Read the model definition and answer for the solid it produces. Units are mm, in the model's axes. Face numbers are marked on the shaded views. A direction names the side the tool comes from. Give positions to 0.01 mm unless a question says otherwise; leave off trailing zeros. Loops run counter-clockwise (first coordinate to the right, second up) from the corner with the lowest first, then second, coordinate; pieces in that order, holes last. Notation, with made-up numbers: (-31, -31.75) -> (-21, -31.75) arc R14 cw to (-21, -21.75) -> close; hole circle Ø4 at (11.5, 76.5). An arc over 180 degrees is marked (long way). Write each question's results on one line, items separated by ' | '. Start each with the question number.
Item 1: Find the intervals of material crossed by line 1 (X direction, y = 23.6, z = 6); line 2 (X direction, y = 23.8, z = 6); line 3 (Y direction, x = -3, z = 9.75), in increasing order.
Item 2: Each of these flat-tipped pins is pushed along its axis until it touches: P1, Ø1.8, axis at x = -26, z = 6, coming from the -Y side; P2, Ø5.5, axis at x = -14.75, y = -19.5, coming from the -Z side; P3, Ø13, axis at y = 10.5, z = 3, coming from the +X side; P4, Ø11, axis at y = -12, z = 5.5, coming from the -X side. Where does it stop, or does it pass through?
Item 3: Section B-B on y = 6 is taken. Write down the section's boundary in (x, z), and give its area (3 significant figures).
Item 4: Section D-D on z = 6 is taken. Write down the section's boundary in (x, y), and give its area (3 significant figures).
Item 5: Section C-C on x = -26 is taken. Write down the section's boundary in (y, z), and give its area (3 significant figures).
Item 6: Which of the six approach directions +Z, -Z, +X, -X, +Y, -Y give full straight-line access (tool end or side, diameter ignored) to the marked faces 1, 2 and 3?
Item 7: Section A-A on z = 18 is taken. Write down the section's boundary in (x, y), and give its area (3 significant figures).
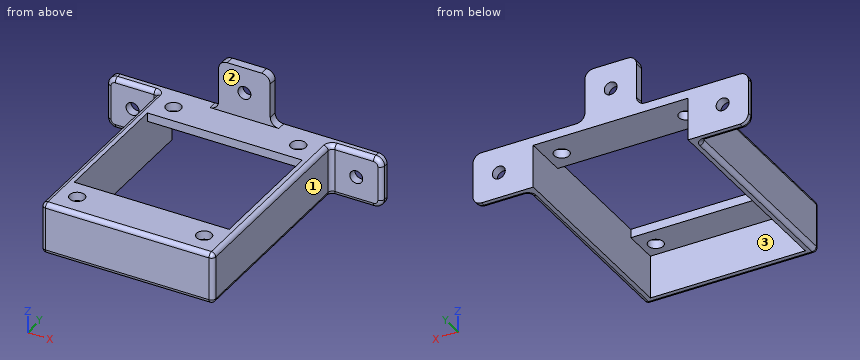
```python
from build123d import *

# Parameters (mm, degrees)
SKETCH_3_W           = 40
SKETCH_3_H           = 50
EXTRUDE_1_DEPTH      = 12
SKETCH_5_W           = 36
SKETCH_5_H           = 46
CUT_EXTRUDE_2_DEPTH  = 10
SKETCH_7_R           = 1.75
CUT_EXTRUDE_6_DEPTH  = 3
SKETCH_11_W          = 12
SKETCH_11_H          = 2
EXTRUDE_2_DEPTH      = 12
FILLET_1_R           = 2
SKETCH_13_R          = 1.5
CUT_EXTRUDE_7_DEPTH  = 2
FILLET_4_R           = 2
SKETCH_14_W          = 12
SKETCH_14_H          = 2
EXTRUDE_3_DEPTH      = 12
FILLET_5_R           = 2
SKETCH_15_R          = 1.5
CUT_EXTRUDE_8_DEPTH  = 12
FILLET_6_R           = 1
FILLET_7_R           = 1
SKETCH_16_W          = 36
SKETCH_16_H          = 10
CUT_EXTRUDE_9_DEPTH  = 63.481997407
SKETCH_19_W          = 36
SKETCH_19_H          = 29.966821032
CUT_EXTRUDE_10_DEPTH = 3


with BuildPart() as part:
    # 草图3 → 凸台-拉伸1 (new body)
    with BuildSketch(Plane.XY):
        Rectangle(SKETCH_3_W, SKETCH_3_H)
    extrude(amount=EXTRUDE_1_DEPTH)

    # 草图5 → 切除-拉伸2 (cut)
    with BuildSketch(Plane(origin=(0, 0, 0), x_dir=(-1, 0, 0), z_dir=(0, 0, -1))):
        Rectangle(SKETCH_5_W, SKETCH_5_H)
    extrude(amount=-CUT_EXTRUDE_2_DEPTH, mode=Mode.SUBTRACT)

    # 草图7 → 切除-拉伸6 (cut)
    with BuildSketch(Plane(origin=(0, 0, 10), x_dir=(-1, 0, 0), z_dir=(0, 0, -1))):
        with Locations((14.5, 19.5)):
            Circle(SKETCH_7_R)
        with Locations((14.75, -19.5)):
            Circle(SKETCH_7_R)
        with Locations((-14.75, -19.5)):
            Circle(SKETCH_7_R)
        with Locations((-14.5, 19.5)):
            Circle(SKETCH_7_R)
    extrude(amount=-CUT_EXTRUDE_6_DEPTH, mode=Mode.SUBTRACT)

    # 草图11 → 凸台-拉伸2 (add)
    with BuildSketch(Plane(origin=(20, 0, 0), x_dir=(0, 0, -1), z_dir=(1, 0, 0))):
        with Locations((-6, 24)):
            Rectangle(SKETCH_11_W, SKETCH_11_H)
    extrude_2 = extrude(amount=EXTRUDE_2_DEPTH)

    # 圆角1
    fillet_1_edges = [part.edges().sort_by_distance(p)[0] for p in [
        (32, 24, 0),
        (32, 24, 12),
    ]]
    fillet(fillet_1_edges, radius=FILLET_1_R)

    # 草图13 → 切除-拉伸7 (cut)
    with BuildSketch(Plane.XZ.offset(-23)):
        with Locations(Location((26, 6, 0), (0, 0, 270))):
            Circle(SKETCH_13_R)
    cut_extrude_7 = extrude(amount=-CUT_EXTRUDE_7_DEPTH, mode=Mode.SUBTRACT)

    # 镜向1: 凸台-拉伸2, 切除-拉伸7 across plane
    add(extrude_2.mirror(Plane(origin=(0, 0, 0), x_dir=(0, 0, 1), z_dir=(1, 0, 0))))
    add(cut_extrude_7.mirror(Plane(origin=(0, 0, 0), x_dir=(0, 0, 1), z_dir=(1, 0, 0))), mode=Mode.SUBTRACT)

    # 圆角4
    fillet_4_edges = [part.edges().sort_by_distance(p)[0] for p in [
        (-32, 24, 0),
        (-32, 24, 12),
    ]]
    fillet(fillet_4_edges, radius=FILLET_4_R)

    # 草图14 → 凸台-拉伸3 (add)
    with BuildSketch(Plane.XY.offset(12)):
        with Locations((0, 24)):
            Rectangle(SKETCH_14_W, SKETCH_14_H)
    extrude(amount=EXTRUDE_3_DEPTH)

    # 圆角5
    fillet_5_edges = [part.edges().sort_by_distance(p)[0] for p in [
        (6, 24, 12),
        (-6, 24, 12),
        (6, 24, 24),
        (-6, 24, 24),
    ]]
    fillet(fillet_5_edges, radius=FILLET_5_R)

    # 草图15 → 切除-拉伸8 (cut)
    with BuildSketch(Plane.XZ.offset(-23)):
        with Locations(Location((0, 18, 0), (0, 0, 270))):
            Circle(SKETCH_15_R)
    extrude(amount=-CUT_EXTRUDE_8_DEPTH, mode=Mode.SUBTRACT)

    # 圆角6
    fillet_6_edges = [part.edges().sort_by_distance(p)[0] for p in [
        (0, -25, 12),
        (0, -25, 0),
        (20, 23, 6),
        (-20, -25, 6),
        (20, -25, 6),
        (-20, 23, 6),
    ]]
    fillet(fillet_6_edges, radius=FILLET_6_R)

    # 圆角7
    # the kernel refuses this fillet: 1 mm, written as the material it takes off along each edge
    with BuildSketch(Plane(origin=(19, -24, 11), x_dir=(1, 0, 0), z_dir=(0, 0, 1))) as fillet_7_piece_1_section:
        Polygon((0, 0), (FILLET_7_R, 0), (FILLET_7_R, -FILLET_7_R), (0, -FILLET_7_R), align=None)
    fillet_7_piece_1 = extrude(amount=FILLET_7_R, mode=Mode.PRIVATE)
    fillet_7_piece_1 = fillet_7_piece_1 - Plane(origin=(19, -24, 11), x_dir=(-0.7071067811865475, 0.7071067811865475, 0), z_dir=(0, 0, 1)) * Sphere(FILLET_7_R, mode=Mode.PRIVATE)
    add(fillet_7_piece_1, mode=Mode.SUBTRACT)
    with BuildSketch(Plane(origin=(19, -24, 1), x_dir=(0, 0, -1), z_dir=(1, 0, 0))) as fillet_7_piece_2_section:
        Polygon((0, 0), (FILLET_7_R, 0), (FILLET_7_R, -FILLET_7_R), (0, -FILLET_7_R), align=None)
    fillet_7_piece_2 = extrude(amount=FILLET_7_R, mode=Mode.PRIVATE)
    fillet_7_piece_2 = fillet_7_piece_2 - Plane(origin=(19, -24, 1), x_dir=(0, 0.7071067811865475, 0.7071067811865475), z_dir=(1, 0, 0)) * Sphere(FILLET_7_R, mode=Mode.PRIVATE)
    add(fillet_7_piece_2, mode=Mode.SUBTRACT)
    with BuildSketch(Plane(origin=(-19, -24, 11), x_dir=(-1, 0, 0), z_dir=(0, 0, 1))) as fillet_7_piece_3_section:
        Polygon((0, 0), (FILLET_7_R, 0), (FILLET_7_R, FILLET_7_R), (0, FILLET_7_R), align=None)
    fillet_7_piece_3 = extrude(amount=FILLET_7_R, mode=Mode.PRIVATE)
    fillet_7_piece_3 = fillet_7_piece_3 - Plane(origin=(-19, -24, 11), x_dir=(0.7071067811865475, 0.7071067811865475, 0), z_dir=(0, 0, 1)) * Sphere(FILLET_7_R, mode=Mode.PRIVATE)
    add(fillet_7_piece_3, mode=Mode.SUBTRACT)
    with BuildSketch(Plane(origin=(-19, -24, 1), x_dir=(0, 0, -1), z_dir=(-1, 0, 0))) as fillet_7_piece_4_section:
        Polygon((0, 0), (FILLET_7_R, 0), (FILLET_7_R, FILLET_7_R), (0, FILLET_7_R), align=None)
    fillet_7_piece_4 = extrude(amount=FILLET_7_R, mode=Mode.PRIVATE)
    fillet_7_piece_4 = fillet_7_piece_4 - Plane(origin=(-19, -24, 1), x_dir=(0, 0.7071067811865475, 0.7071067811865475), z_dir=(-1, 0, 0)) * Sphere(FILLET_7_R, mode=Mode.PRIVATE)
    add(fillet_7_piece_4, mode=Mode.SUBTRACT)
    with BuildSketch(Plane(origin=(-32, 23, 10), x_dir=(1, 0, 0), z_dir=(0, 0, -1))) as fillet_7_piece_5:
        with BuildLine():
            CenterArc((FILLET_7_R, -FILLET_7_R), FILLET_7_R, 90, 90)
            Line((0, -FILLET_7_R), (0, 0))
            Line((0, 0), (FILLET_7_R, 0))
        make_face()
    extrude(amount=8, mode=Mode.SUBTRACT)
    with BuildSketch(Plane(origin=(-21, 23, 12), x_dir=(0, 1, 0), z_dir=(-1, 0, 0)), Plane(origin=(-21, 23, 0), x_dir=(0, 0, 1), z_dir=(-1, 0, 0))) as fillet_7_piece_6:
        with BuildLine():
            CenterArc((FILLET_7_R, FILLET_7_R), FILLET_7_R, 180, 90)
            Line((0, FILLET_7_R), (0, 0))
            Line((0, 0), (FILLET_7_R, 0))
        make_face()
    extrude(amount=9, mode=Mode.SUBTRACT)
    with BuildSketch(Plane(origin=(-30, 23, 10), x_dir=(0, 0, 1), z_dir=(1, 0, 0))) as fillet_7_piece_7:
        with BuildLine():
            CenterArc((2 - FILLET_7_R, -FILLET_7_R), FILLET_7_R, 0, 90)
            Line((2, -FILLET_7_R), (2, 0))
            Line((2, 0), (2 - FILLET_7_R, 0))
        make_face()
    revolve(axis=Axis((-30, 23, 10), (0, -1, 0)), revolution_arc=90, mode=Mode.SUBTRACT)
    with BuildSketch(Plane(origin=(-30, 23, 2), x_dir=(-1, 0, 0), z_dir=(0, 0, 1))) as fillet_7_piece_8:
        with BuildLine():
            CenterArc((2 - FILLET_7_R, -FILLET_7_R), FILLET_7_R, 0, 90)
            Line((2, -FILLET_7_R), (2, 0))
            Line((2, 0), (2 - FILLET_7_R, 0))
        make_face()
    revolve(axis=Axis((-30, 23, 2), (0, -1, 0)), revolution_arc=90, mode=Mode.SUBTRACT)
    with BuildSketch(Plane(origin=(-20, -24, 12), x_dir=(1, 0, 0), z_dir=(0, 1, 0)), Plane(origin=(-20, -24, 0), x_dir=(0, 0, 1), z_dir=(0, 1, 0)), Plane(origin=(20, 22, 12), x_dir=(-1, 0, 0), z_dir=(0, -1, 0)), Plane(origin=(20, 22, 0), x_dir=(0, 0, 1), z_dir=(0, -1, 0))) as fillet_7_piece_9:
        with BuildLine():
            CenterArc((FILLET_7_R, FILLET_7_R), FILLET_7_R, 180, 90)
            Line((0, FILLET_7_R), (0, 0))
            Line((0, 0), (FILLET_7_R, 0))
        make_face()
    extrude(amount=46, mode=Mode.SUBTRACT)
    with BuildSketch(Plane(origin=(-21, 22, 0), x_dir=(1, 0, 0), z_dir=(0, -1, 0))) as fillet_7_piece_10:
        with BuildLine():
            CenterArc((1 + FILLET_7_R, FILLET_7_R), FILLET_7_R, 180, 90)
            Line((1 + FILLET_7_R, 0), (1, 0))
            Line((1, 0), (1, FILLET_7_R))
        make_face()
    revolve(axis=Axis((-21, 22, 0), (0, 0, 1)), revolution_arc=90, mode=Mode.SUBTRACT)
    with BuildSketch(Plane(origin=(-21, 22, 12), x_dir=(1, 0, 0), z_dir=(0, -1, 0))) as fillet_7_piece_11:
        with BuildLine():
            CenterArc((1 + FILLET_7_R, -FILLET_7_R), FILLET_7_R, 90, 90)
            Line((1, -FILLET_7_R), (1, 0))
            Line((1, 0), (1 + FILLET_7_R, 0))
        make_face()
    revolve(axis=Axis((-21, 22, 12), (0, 0, 1)), revolution_arc=90, mode=Mode.SUBTRACT)
    with BuildSketch(Plane(origin=(21, 22, 0), x_dir=(0, 1, 0), z_dir=(1, 0, 0))) as fillet_7_piece_12:
        with BuildLine():
            CenterArc((1 + FILLET_7_R, FILLET_7_R), FILLET_7_R, 180, 90)
            Line((1 + FILLET_7_R, 0), (1, 0))
            Line((1, 0), (1, FILLET_7_R))
        make_face()
    revolve(axis=Axis((21, 22, 0), (0, 0, 1)), revolution_arc=90, mode=Mode.SUBTRACT)
    with BuildSketch(Plane(origin=(21, 22, 12), x_dir=(0, 1, 0), z_dir=(1, 0, 0))) as fillet_7_piece_13:
        with BuildLine():
            CenterArc((1 + FILLET_7_R, -FILLET_7_R), FILLET_7_R, 90, 90)
            Line((1, -FILLET_7_R), (1, 0))
            Line((1, 0), (1 + FILLET_7_R, 0))
        make_face()
    revolve(axis=Axis((21, 22, 12), (0, 0, 1)), revolution_arc=90, mode=Mode.SUBTRACT)
    with BuildSketch(Plane(origin=(32, 23, 10), x_dir=(-1, 0, 0), z_dir=(0, 0, -1))) as fillet_7_piece_14:
        with BuildLine():
            CenterArc((FILLET_7_R, FILLET_7_R), FILLET_7_R, 180, 90)
            Line((0, FILLET_7_R), (0, 0))
            Line((0, 0), (FILLET_7_R, 0))
        make_face()
    extrude(amount=8, mode=Mode.SUBTRACT)
    with BuildSketch(Plane(origin=(21, 23, 0), x_dir=(0, 0, 1), z_dir=(1, 0, 0)), Plane(origin=(21, 23, 12), x_dir=(0, 1, 0), z_dir=(1, 0, 0))) as fillet_7_piece_15:
        with BuildLine():
            CenterArc((FILLET_7_R, -FILLET_7_R), FILLET_7_R, 90, 90)
            Line((0, -FILLET_7_R), (0, 0))
            Line((0, 0), (FILLET_7_R, 0))
        make_face()
    extrude(amount=9, mode=Mode.SUBTRACT)
    with BuildSketch(Plane(origin=(30, 23, 2), x_dir=(0, 0, -1), z_dir=(-1, 0, 0))) as fillet_7_piece_16:
        with BuildLine():
            CenterArc((2 - FILLET_7_R, -FILLET_7_R), FILLET_7_R, 0, 90)
            Line((2, -FILLET_7_R), (2, 0))
            Line((2, 0), (2 - FILLET_7_R, 0))
        make_face()
    revolve(axis=Axis((30, 23, 2), (0, -1, 0)), revolution_arc=90, mode=Mode.SUBTRACT)
    with BuildSketch(Plane(origin=(30, 23, 10), x_dir=(1, 0, 0), z_dir=(0, 0, -1))) as fillet_7_piece_17:
        with BuildLine():
            CenterArc((2 - FILLET_7_R, -FILLET_7_R), FILLET_7_R, 0, 90)
            Line((2, -FILLET_7_R), (2, 0))
            Line((2, 0), (2 - FILLET_7_R, 0))
        make_face()
    revolve(axis=Axis((30, 23, 10), (0, -1, 0)), revolution_arc=90, mode=Mode.SUBTRACT)

    # 草图16 → 切除-拉伸9 (cut, through all)
    with BuildSketch(Plane(origin=(0, 23, 0), x_dir=(-1, 0, 0), z_dir=(0, -1, 0))):
        with Locations((0, -5)):
            Rectangle(SKETCH_16_W, SKETCH_16_H)
    extrude(amount=-CUT_EXTRUDE_9_DEPTH, mode=Mode.SUBTRACT)

    # 草图19 → 切除-拉伸10 (cut)
    with BuildSketch(Plane.XY.offset(12)):
        Rectangle(SKETCH_19_W, SKETCH_19_H)
    extrude(amount=-CUT_EXTRUDE_10_DEPTH, mode=Mode.SUBTRACT)


solid = part.part
```
Findings:
1) line 1: -31.92 to -27.5, -24.5 to -18, 18 to 24.5, 27.5 to 31.92 | line 2: -31.98 to -27.5, -24.5 to -18, 18 to 24.5, 27.5 to 31.98 | line 3: -25 to -23
2) P1: through | P2: z = 10 | P3: x = 20 | P4: x = -20
3) outline: (-20, 1) arc R1 ccw to (-19, 0) -> (-18, 0) -> (-18, 12) -> (-19, 12) arc R1 ccw to (-20, 11) -> close; (18, 0) -> (19, 0) arc R1 ccw to (20, 1) -> (20, 11) arc R1 ccw to (19, 12) -> (18, 12) -> close | area: 47.1 mm2
4) outline: (-32, 24) arc R1 ccw to (-31, 23) -> (-27.5, 23) -> (-27.5, 25) -> (-32, 25) -> close; (-24.5, 23) -> (-21, 23) arc R1 cw to (-20, 22) -> (-20, -24) arc R1 ccw to (-19, -25) -> (19, -25) arc R1 ccw to (20, -24) -> (20, 22) arc R1 cw to (21, 23) -> (24.5, 23) -> (24.5, 25) -> (18, 25) -> (18, -23) -> (-18, -23) -> (-18, 25) -> (-24.5, 25) -> close; (27.5, 23) -> (31, 23) arc R1 ccw to (32, 24) -> (32, 25) -> (27.5, 25) -> close | area: 308 mm2
5) outline: (23, 1) arc R1 ccw to (24, 0) -> (25, 0) -> (25, 4.5) -> (23, 4.5) -> close; (23, 7.5) -> (25, 7.5) -> (25, 12) -> (24, 12) arc R1 ccw to (23, 11) -> close | area: 17.6 mm2
6) face 1: +Z, -Z, +X, -Y | face 2: +Z, +X, -X, -Y | face 3: -Z, +Y
7) outline: (-6, 23) -> (-1.5, 23) -> (-1.5, 25) -> (-6, 25) -> close; (1.5, 23) -> (6, 23) -> (6, 25) -> (1.5, 25) -> close | area: 18.0 mm2
